Source: CAD feature listing. Evaluate the final solid. Frame: model axes, mm. A direction names the side the tool comes from. Round coordinates to 2 decimals unless told otherwise and drop trailing zeros. Write each loop counter-clockwise with the first axis right and the second up, starting at its lowest first coordinate (ties: lowest second). Pieces come first, ordered by that corner, then holes. Notation, with made-up numbers: M 64.25,-36.75 L 118.25,-36.75 A13 ccw 118.25,-20.75 Z; hole C 61,63 d3. An arc over 180 degrees is marked long. Put each result on its own line as item: value. Start each with the question number.
```python
from build123d import *

# Parameters (mm, degrees)
CYLINDER001_R     = 2
CYLINDER001_DEPTH = 30
ARRAY_COUNT       = 8
CYLINDER_R        = 15
CYLINDER_DEPTH    = 20
CHAMFER_SIZE      = 1.6


with BuildPart() as array:
    # Cylinder001 → Cylinder001 (new body)
    with BuildSketch(Plane(origin=(14, 0, 0), x_dir=(1, 0, 0), z_dir=(0, 0, 1))):
        Circle(CYLINDER001_R)
    extrude(amount=CYLINDER001_DEPTH)

    # Array: Array ×8 about axis
    array_axis = Axis((0, 0, 0), (0, 0, 1))


with BuildPart() as array_1:
    add(array.part)
    for i in range(1, ARRAY_COUNT):
        add(array.part.rotate(array_axis, i * 360 / ARRAY_COUNT))


with BuildPart() as array_2:
    # Array placement: moved
    add(array_1.part.moved(Location((0, 0, 7))))


with BuildPart() as cut:
    # Cylinder → Cylinder (new body)
    with BuildSketch(Plane.XY):
        Circle(CYLINDER_R)
    extrude(amount=CYLINDER_DEPTH)

    # Chamfer
    chamfer_edges = [cut.edges().sort_by_distance(p)[0] for p in [
        (-15, 0, 20),
    ]]
    chamfer(chamfer_edges, length=CHAMFER_SIZE)

    # Cut: cut Array
    add(array_2.part, mode=Mode.SUBTRACT)


solid = cut.part
```
(1) Section query D-D (z = 5). Return loops of the section in (x, y), and give its area (3 significant figures).
(2) Ray query, line 1 along Z through (x, y) = (-13.5, -1); line 2 along X through (y, z) = (13.5, 13.75); line 3 along X through (y, z) = (0, 12). Return the intervals inside material, ascending.
(3) Section query A-A (z = 16.25). Return loops of the section in (x, y).
(4) Access query for faces 5 (the conical face through (-13.09, 5.48, 19.21)), 6 (the cylindrical face through (-8.526, 8.446, 13.409)). Directions: +Z, -Z, +X, -X, +Y, -Y. A direction counts if a zero-diameter tool reaches every point of the face in a straight line with its end or side. Return the directions, or none.
(5) Pull-direction query (Y, two-part tool) for faces 1 (the conical face through (-5.38, 13.13, 19.21)), 2 (the cylindrical face through (8.446, 8.526, 13.409)), 3 (the cylindrical face through (13.856, -5.745, 9.071)), 4 (the conical face through (-5.48, -13.09, 19.21)); classes: +Y half, -Y half, draft (parallel to the pull), parting line (faces both ways), or undercut.
(6) Section query C-C (y = 0.75). Return loops of the section in (x, z).
(7) Contact query for flat-ended pins moving along their axis: P1, Ø1.9, axis at x = 10.5, y = 10, coming from the +Z side; P2, Ø2, axis at y = 6, z = 9, coming from the +X side; P3, Ø1.5, axis at x = -10.5, z = 15.5, coming from the +Y side. Output: stop coordinate, or through.
(8) Section query B-B (x = 0). Return loops of the section in (y, z), and give its area (3 significant figures).
Entries:
1. outline: C 0,0 d30
1. area: 707 mm2
2. line 1: 0 to 7
2. line 2: -6.54 to -1.94, 1.94 to 6.54
2. line 3: -12 to 12
3. outline: M -14.89,-1.79 A15 ccw -11.8,-9.27 A2 cw long -9.27,-11.8 A15 ccw -1.79,-14.89 A2 cw long 1.79,-14.89 A15 ccw 9.27,-11.8 A2 cw long 11.8,-9.27 A15 ccw 14.89,-1.79 A2 cw long 14.89,1.79 A15 ccw 11.8,9.27 A2 cw long 9.27,11.8 A15 ccw 1.79,14.89 A2 cw long -1.79,14.89 A15 ccw -9.27,11.8 A2 cw long -11.8,9.27 A15 ccw -14.89,1.79 A2 cw long Z
4. face 5: +Z, -X, +Y
4. face 6: +Z
5. face 1: +Y half
5. face 2: undercut
5. face 3: parting line
5. face 4: -Y half
6. outline: M -14.98,0 L 14.98,0 L 14.98,7 L 12.15,7 L 12.15,20 L -12.15,20 L -12.15,7 L -14.98,7 Z
7. P1: z = 7
7. P2: x = 14.14
7. P3: y = 8.42
8. outline: M -15,0 L 15,0 L 15,7 L 12,7 L 12,20 L -12,20 L -12,7 L -15,7 Z
8. area: 522 mm2
